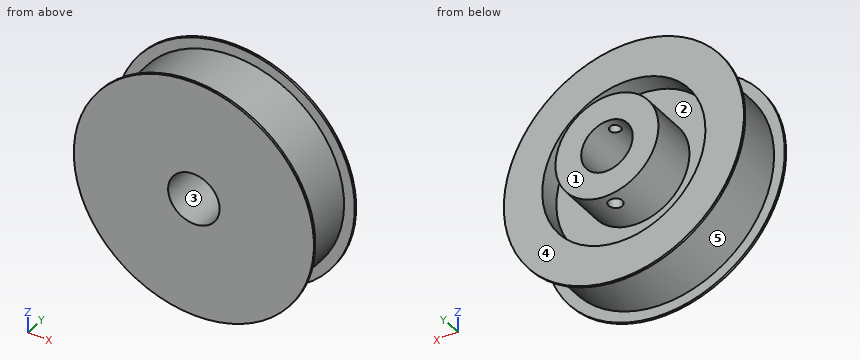
from build123d import *

# Parameters (mm, degrees)
CROQUIS1_R                                     = 25.465
SALIENTE_EXTRUIR1_DEPTH                        = 7.5
CROQUIS2_R                                     = 27.965
SALIENTE_EXTRUIR2_DEPTH                        = 0.5
SALIENTE_EXTRUIR3_START                        = -14.5
CROQUIS2_2_R                                   = 27.965
SALIENTE_EXTRUIR3_DEPTH                        = 0.5
CROQUIS3_R                                     = 19
SALIENTE_EXTRUIR4_DEPTH                        = 21
CORTAR_EXTRUIR1_DEPTH                          = 45.545846608
CORTAR_EXTRUIR1_DEPTH_BACK                     = 45.545846608
CROQUIS4_R                                     = 6
CORTAR_EXTRUIR2_START                          = -11
CROQUIS5_R                                     = 19
CROQUIS5_R_2                                   = 12
CORTAR_EXTRUIR2_DEPTH                          = 11
PERFORADOR_PARA_ROSCAR_PARA_MACHO_DE_ROS_REACH = 60.109
PERFORADOR_PARA_ROSCAR_PARA_MACHO_DE_2_R       = 1.25
TALADRO_DE_MARGEN_PARA_M32_REACH               = 52.611
TALADRO_DE_MARGEN_PARA_M32_BORE_R              = 1.6


with BuildPart() as part:
    # Croquis1 → Saliente-Extruir1 (new, symmetric)
    with BuildSketch(Plane(origin=(0, 0, 0), x_dir=(-1, 0, 0), z_dir=(0, 1, 0))):
        with Locations(Location((0, 0, 0), (0, 0, 90))):
            Circle(CROQUIS1_R)
    extrude(amount=SALIENTE_EXTRUIR1_DEPTH, both=True)

    # Croquis2 → Saliente-Extruir2 (add)
    with BuildSketch(Plane(origin=(0, 7.5, 0), x_dir=(-1, 0, 0), z_dir=(0, 1, 0))):
        with Locations(Location((0, 0, 0), (0, 0, 90))):
            Circle(CROQUIS2_R)
    extrude(amount=-SALIENTE_EXTRUIR2_DEPTH)

    # Croquis2<2> → Saliente-Extruir3 (add)
    with BuildSketch(Plane(origin=(0, 7.5, 0), x_dir=(-1, 0, 0), z_dir=(0, 1, 0)).offset(SALIENTE_EXTRUIR3_START)):
        with Locations(Location((0, 0, 0), (0, 0, 90))):
            Circle(CROQUIS2_2_R)
    extrude(amount=-SALIENTE_EXTRUIR3_DEPTH)

    # Croquis3 → Saliente-Extruir4 (add)
    with BuildSketch(Plane(origin=(0, -7.5, 0), x_dir=(-1, 0, 0), z_dir=(0, 1, 0))):
        with Locations(Location((0, 0, 0), (0, 0, 270))):
            Circle(CROQUIS3_R)
    extrude(amount=SALIENTE_EXTRUIR4_DEPTH)

    # Croquis4 → Cortar-Extruir1 (cut, two sides: drawn at the far end of the back side and taken through both)
    with BuildSketch(Plane(origin=(0, -7, 0), x_dir=(-1, 0, 0), z_dir=(0, 1, 0)).offset(-CORTAR_EXTRUIR1_DEPTH_BACK)):
        with Locations(Location((0, 0, 0), (0, 0, 90))):
            Circle(CROQUIS4_R)
    extrude(amount=CORTAR_EXTRUIR1_DEPTH + CORTAR_EXTRUIR1_DEPTH_BACK, mode=Mode.SUBTRACT)

    # Croquis5 → Cortar-Extruir2 (cut)
    with BuildSketch(Plane(origin=(0, 13.5, 0), x_dir=(-1, 0, 0), z_dir=(0, 1, 0)).offset(CORTAR_EXTRUIR2_START)):
        with Locations(Location((0, 0, 0), (0, 0, 90))):
            Circle(CROQUIS5_R)
        with Locations(Location((0, 0, 0), (0, 0, 90))):
            Circle(CROQUIS5_R_2, mode=Mode.SUBTRACT)
    extrude(amount=CORTAR_EXTRUIR2_DEPTH, mode=Mode.SUBTRACT)

    # Perforador para roscar para macho de 2 → Perforador para roscar para macho de roscar para M31 (cut, up to next)
    with BuildSketch(Plane(origin=(-12, 0, 12), x_dir=(0, 1, 0), z_dir=(0, 0, 1)), mode=Mode.PRIVATE) as perforador_para_roscar_para_macho_de_ros_sk1:
        with Locations((10.5, -12)):
            Circle(PERFORADOR_PARA_ROSCAR_PARA_MACHO_DE_2_R)
    perforador_para_roscar_para_macho_de_ros_tool1 = extrude(perforador_para_roscar_para_macho_de_ros_sk1.sketch, amount=-PERFORADOR_PARA_ROSCAR_PARA_MACHO_DE_ROS_REACH, mode=Mode.PRIVATE) & part.part
    add(perforador_para_roscar_para_macho_de_ros_tool1.solids().sort_by_distance((0, 10.5, 12))[0], mode=Mode.SUBTRACT)

    # Taladro de margen para M32 bore → Taladro de margen para M32 (cut, up to next)
    with BuildSketch(Plane(origin=(0, 0, -12), x_dir=(-1, 0, 0), z_dir=(0, 0, -1)), mode=Mode.PRIVATE) as taladro_de_margen_para_m32_sk1:
        with Locations((0, 10.5)):
            Circle(TALADRO_DE_MARGEN_PARA_M32_BORE_R)
    taladro_de_margen_para_m32_tool1 = extrude(taladro_de_margen_para_m32_sk1.sketch, amount=-TALADRO_DE_MARGEN_PARA_M32_REACH, mode=Mode.PRIVATE) & part.part
    add(taladro_de_margen_para_m32_tool1.solids().sort_by_distance((0, 10.5, -12))[0], mode=Mode.SUBTRACT)


solid = part.part
Geometry: final body of the model. Coordinates: model frame, mm. Face numbers are marked on the shaded views. A direction names the side the tool comes from. Round coordinates to 2 decimals unless told otherwise and drop trailing zeros. Order: outer loops, then holes, each group sorted by start corner. A loop starts at its lowest first (then second) coordinate and runs counter-clockwise, first axis right, second up. Notation, with made-up numbers: (-24, 29) -> (-13, 29) arc R28 cw to (-13, 58) -> close; hole circle Ø2 at (-0.5, -8.75). An arc over 180 degrees is marked (long way). Put each result on its own line as item: value. Start each with the question number.
Q1. Pull-direction query (X, two-part tool) for the marked faces 3, 4 and 5; classes: +X half, -X half, draft (parallel to the pull), parting line (faces both ways), or undercut.
Q2. Section C-C on y = 10.5. Return the cut outline in (x, z), and give its area (3 significant figures).
Q3. First-contact query: pin 1 (1.5 mm diameter, centred on x = 6, z = 21, fed in from +Y); pin 2 (5 mm diameter, centred on x = -10.5, y = -5, fed in from +Z); pin 3 (3 mm diameter, centred on y = 7.5, z = -19, fed in from +X). Flat tips, straight axial feed; report the tip coordinate or a pass-through.
Q4. Section D-D on x = 13.5. Return the cut outline in (y, z), and give its area (3 significant figures).
Q5. Line query: probe 1 along X at (y, z) = (6, 0) (3 decimals); probe 2 along Y at (x, z) = (0, -10.25); probe 3 along Z at (x, y) = (0, 8.75). Output: solid intervals per line, ascending.
Q6. Section B-B on z = 0. Return the cut outline in (x, y) (3 decimals), and give its area (3 significant figures).
Q7. Section A-A on y = 4.25. Return the cut outline in (x, z) (3 decimals).
Q8. Reachability of the marked faces 1 and 2 from +Z, -Z, +X, -X, +Y, -Y: full face, straight path, thin tool, end or side. Return the list, or none.
Ans:
1. face 3: undercut
1. face 4: draft
1. face 5: parting line
2. outline: (-1.6, -11.89) -> (-1.6, -5.78) arc R6 cw to (-1.25, 5.87) -> (-1.25, 11.93) arc R12 ccw to start; (1.25, 5.87) arc R6 cw to (1.6, -5.78) -> (1.6, -11.89) arc R12 ccw to (1.25, 11.93) -> close
2. area: 305 mm2
3. pin 1: stops at y = 7.5
3. pin 2: stops at z = 26.48
3. pin 3: stops at x = 21.81
4. outline: (-7.5, -24.49) -> (-7, -24.49) -> (-7, -21.59) -> (7, -21.59) -> (7, -24.49) -> (7.5, -24.49) -> (7.5, -13.37) -> (2.5, -13.37) -> (2.5, 13.37) -> (7.5, 13.37) -> (7.5, 24.49) -> (7, 24.49) -> (7, 21.59) -> (-7, 21.59) -> (-7, 24.49) -> (-7.5, 24.49) -> close
4. area: 520 mm2
5. probe 1: x = -25.465 to -19, -12 to -6, 6 to 12, 19 to 25.465
5. probe 2: y = -7.5 to 8.9, 12.1 to 13.5
5. probe 3: z = -12 to -6, 6 to 12
6. outline: (-27.965, -7.5) -> (-6, -7.5) -> (-6, 13.5) -> (-12, 13.5) -> (-12, 2.5) -> (-19, 2.5) -> (-19, 7.5) -> (-27.965, 7.5) -> (-27.965, 7) -> (-25.465, 7) -> (-25.465, -7) -> (-27.965, -7) -> close; (6, -7.5) -> (27.965, -7.5) -> (27.965, -7) -> (25.465, -7) -> (25.465, 7) -> (27.965, 7) -> (27.965, 7.5) -> (19, 7.5) -> (19, 2.5) -> (12, 2.5) -> (12, 13.5) -> (6, 13.5) -> close
6. area: 591 mm2
7. outline: circle Ø50.93 at (0, 0); circle Ø24 at (0, 0); hole circle Ø38 at (0, 0); hole circle Ø12 at (0, 0)
8. face 1: +Z, -Z, +X, -X, +Y
8. face 2: +Y
